from build123d import *

# Parameters (mm, degrees)
F1_DEPTH = 76.2
F2_R     = 12.7
F3_R     = 7.921290647
F4_DEPTH = 101.6


# Not quite as in the source:
# - a feature names something its author has since deleted; it is built from what else it names


with BuildPart() as f1:
    # F0 (on Front) → F1 (new body)
    with BuildSketch(Plane.XZ):
        with BuildLine():
            Line((25.4, -25.4), (25.4, 0))
            ThreePointArc((25.4, 0), (0, 25.4), (-25.4, 0))
            Line((-25.4, 0), (-25.4, -25.4))
            Line((-25.4, -25.4), (-63.5, -25.4))
            Line((-63.5, -25.4), (-63.5, -35.56))
            Line((-63.5, -35.56), (63.5, -35.56))
            Line((63.5, -35.56), (63.5, -25.4))
            Line((63.5, -25.4), (25.4, -25.4))
        make_face()
    extrude(amount=F1_DEPTH)

    # F2
    f2_edges = [f1.edges().sort_by_distance(p)[0] for p in [
        (25.4, -38.1, -25.4),
        (-25.4, -38.1, -25.4),
    ]]
    fillet(f2_edges, radius=F2_R)

    # F3 (on face) → F4 (cut)
    with BuildSketch(Plane.XZ.offset(76.2)):
        Circle(F3_R)
    extrude(amount=-F4_DEPTH, mode=Mode.SUBTRACT)


solid = f1.part
Can you work these out from the model? Positions are in its coordinate system, mm. A direction names the side the tool comes from. Give positions to 0.01 mm unless a question says otherwise; leave off trailing zeros. Order: outer loops, then holes, each group sorted by start corner. A loop starts at its lowest first (then second) coordinate and runs counter-clockwise, first axis right, second up. Notation, with made-up numbers: M 2,-14.5 L 27,-14.5 A23 ccw 27,20.5 Z; hole C -37,6 d8. An arc over 180 degrees is marked long. Use a Markdown table: item, result. Add a question column.
Item 1: If I drill on L1, parallel to Z at x = 53.5, y = -19.5; L2, parallel to Z at x = 0, y = -27.5; L3, parallel to X at y = -25, z = -11, over which ranges is the centre line in solid material (lowest first)? Write a range as [from, to].
Item 2: We'd pull the mould along Z, two halves only. Please class faces 4 (the flat face through (-63.5, -38, -30)), 5 (the cylindrical face through (-1.031, -38.633, 7.854)), 6 (the flat face through (-1, -38, -35.56)): +Z half, -Z half, draft (parallel to the pull), parting line (faces both ways), or undercut.
Item 3: Suppose I cut it at A-A (x = 0). List the corners of the cut face in (y, z) for me, then the cut area to 3 significant figures.
Item 4: For faces 1 (the flat face through (-1, 0, -11)), 2 (the flat face through (-51, -38, -25.4)), 3 (the flat face through (25.4, -38, -6)), which set-ups out of +Z, -Z, +X, -X, +Y, -Y let a thin tool reach every point of the face, with its end or its side?
Item 5: Will these pins go through, and if not, where does the flat tip stop? pin 1 (8 mm diameter, centred on y = -34, z = 3.5, fed in from +X); pin 2 (20.5 mm diameter, centred on x = -47.5, y = -37.5, fed in from +Z); pin 3 (14 mm diameter, centred on y = -49, z = -9.5, fed in from -X).
Item 6: Suppose I cut it at D-D (x = 46). List the corners of the cut face in (y, z) for me, then the cut area to 3 significant figures.
Item 7: Suppose I cut it at C-C (z = 3). List the corners of the cut face in (x, y) for me.
Item 8: Suppose I cut it at B-B (y = -9). List the corners of the cut face in (x, z) for me, then the cut area to 3 significant figures.
Answer sheet:
| question | item | result |
|---|---|---|
| 1 | L1 | z = [-35.56, -25.4] |
| 1 | L2 | z = [-35.56, -7.92], [7.92, 25.4] |
| 1 | L3 | x = [-25.4, 25.4] |
| 2 | face 4 | draft |
| 2 | face 5 | undercut |
| 2 | face 6 | -Z half |
| 3 | outline | M -76.2,-35.56 L 0,-35.56 L 0,-7.92 L -76.2,-7.92 Z; M -76.2,7.92 L 0,7.92 L 0,25.4 L -76.2,25.4 Z |
| 3 | area | 3,440 mm² |
| 4 | face 1 | +Z, -Z, +X, -X, +Y |
| 4 | face 2 | +Z, -X, +Y, -Y |
| 4 | face 3 | +Z, +X, +Y, -Y |
| 5 | pin 1 | stops at x = 25.4 |
| 5 | pin 2 | stops at z = -25.37 |
| 5 | pin 3 | stops at x = -25.98 |
| 6 | outline | M -76.2,-35.56 L 0,-35.56 L 0,-25.4 L -76.2,-25.4 Z |
| 6 | area | 774 mm² |
| 7 | outline | M -25.22,-76.2 L -7.33,-76.2 L -7.33,0 L -25.22,0 Z; M 7.33,-76.2 L 25.22,-76.2 L 25.22,0 L 7.33,0 Z |
| 8 | outline | M -63.5,-35.56 L 63.5,-35.56 L 63.5,-25.4 L 38.1,-25.4 A12.7 cw 25.4,-12.7 L 25.4,0 A25.4 ccw -25.4,0 L -25.4,-12.7 A12.7 cw -38.1,-25.4 L -63.5,-25.4 Z; hole C 0,0 d15.84 |
| 8 | area | 3,470 mm² |
